Could you check a few things on this drawing? It's one solid part, dimensions in mm from its lowest x, y, z. A direction names the side the tool comes from. Give positions to 0.01 mm unless a question says otherwise; leave off trailing zeros. Loops run counter-clockwise (first coordinate to the right, second up) from the corner with the lowest first, then second, coordinate; pieces in that order, holes last. Notation, with made-up numbers: (-7.75, 66) -> (-0.75, 66) arc R32 cw to (-0.75, 93) -> close; hole circle Ø4 at (69.5, -40). An arc over 180 degrees is marked (long way). Use CSV: the item, a comma, the result in double quotes.
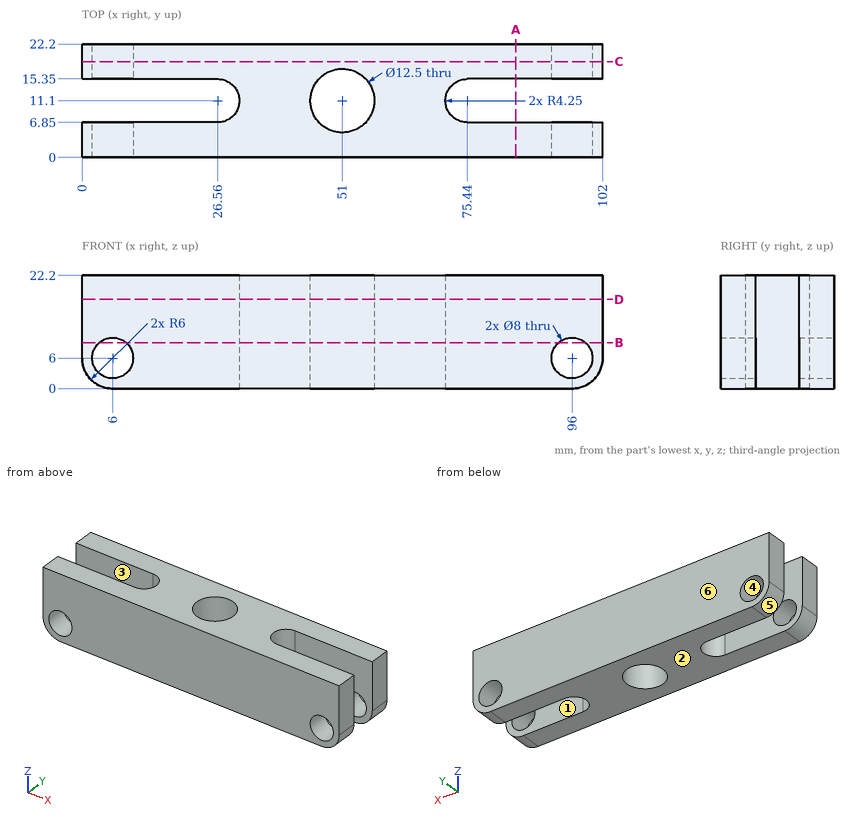
(1) If we section it at A-A, the plane x = 85: Write out the boundary of the cut face in (y, z), then the cut area to 3 significant figures.
Answer sheet:
outline,"(0, 0) -> (6.85, 0) -> (6.85, 22.2) -> (0, 22.2) -> close; (15.35, 0) -> (22.2, 0) -> (22.2, 22.2) -> (15.35, 22.2) -> close"
area,"304 mm2"
(2) Which directions (+Z, -Z, +X, -X, +Y, -Y) give clear straight access to the entire face, cutting with the end or side of a thin tool? Please do the marked faces 1, 2 and 3.
Answer sheet:
face 1,"+Z, -Z, +X"
face 2,"-Z, +X, -X, +Y, -Y"
face 3,"+Z, -Z, -X"
(3) Will these pins go through, and if not, where does the flat tip stop? pin 1 Ø7 at (x, z) = (6, 6) entering from +Y; pin 2 Ø1 at (y, z) = (11, 17) entering from -X; pin 3 Ø10.5 at (x, z) = (6, 6) entering from -Y; pin 4 Ø2 at (y, z) = (13.5, 16.5) entering from -X.
Answer sheet:
pin 1,"passes through"
pin 2,"stops at x = 30.77"
pin 3,"stops at y = 0"
pin 4,"stops at x = 29.11"
(4) If we section it at C-C, the plane y = 18.75: Write out the boundary of the cut face in (x, z).
Answer sheet:
outline,"(0, 6) arc R6 ccw to (6, 0) -> (96, 0) arc R6 ccw to (102, 6) -> (102, 22.2) -> (0, 22.2) -> close; hole circle Ø8 at (6, 6); hole circle Ø8 at (96, 6)"
(5) If we section it at D-D, the plane z = 17.5: Write out the boundary of the cut face in (x, y), then the cut area to 3 significant figures.
Answer sheet:
outline,"(0, 0) -> (102, 0) -> (102, 6.85) -> (75.44, 6.85) arc R4.25 cw to (75.44, 15.35) -> (102, 15.35) -> (102, 22.2) -> (0, 22.2) -> (0, 15.35) -> (26.56, 15.35) arc R4.25 cw to (26.56, 6.85) -> (0, 6.85) -> close; hole circle Ø12.5 at (51, 11.1)"
area,"1,630 mm2"
(6) If we section it at B-B, the plane z = 9: Give the number of separate pieces and of enclosed holes in the cut face, then the cut area to 3 significant figures.
Answer sheet:
separate pieces,"5"
enclosed holes,"1"
area,"1,490 mm2"
(7) We'd pull the mould along X, two halves only. Please class the marked faces 4, 5 and 6: released by +X, released by -X, zero draft, split by the parting line, or undercut.
Answer sheet:
face 4,"undercut"
face 5,"released by -X"
face 6,"zero draft"
(8) If I drill on L1, parallel to X at y = 4.75, z = 6; L2, parallel to Y at x = 18.5, z = 2.75; L3, parallel to Z at x = 6, y = 5.25, over which ranges is the centre line in solid material (lowest first)? Write a range as from..to.
Answer sheet:
L1,"x = 0..2, 10..92, 100..102"
L2,"y = 0..6.85, 15.35..22.2"
L3,"z = 0..2, 10..22.2"
